Work out the finished part from the listing and answer in its coordinate system (mm). Give positions to 0.01 mm unless a question says otherwise; leave off trailing zeros. Order: outer loops, then holes, each group sorted by start corner. A loop starts at its lowest first (then second) coordinate and runs counter-clockwise, first axis right, second up. Notation, with made-up numbers: (13.25, 59.5) - (70.25, 59.5) arc R27 cw to (70.25, 76.5) - close; hole circle Ø1 at (59, 41.25). An arc over 180 degrees is marked (long way). Write each question's results on one line, items separated by ' | '.
from build123d import *

# Parameters (mm, degrees)
SKETCH1_W           = 165.75
SKETCH1_H           = 75
BOSS_EXTRUDE1_DEPTH = 3
SKETCH2_W           = 151.75
SKETCH2_H           = 5
CUT_EXTRUDE1_DEPTH  = 183.692731916
FILLET4_R           = 1
FILLET5_R           = 1
FILLET6_R           = 1
FILLET7_R           = 1
FILLET8_R           = 1
FILLET9_R           = 1
FILLET10_R          = 1
FILLET11_R          = 1
FILLET12_R          = 1
FILLET13_R          = 1
FILLET14_R          = 1
FILLET15_R          = 1
FILLET16_R          = 1
FILLET17_R          = 1
FILLET18_R          = 1
FILLET19_R          = 1
FILLET20_R          = 1
FILLET21_R          = 1
FILLET22_R          = 1
FILLET23_R          = 1
FILLET24_R          = 1
FILLET25_R          = 1
FILLET26_R          = 1
FILLET27_R          = 1


with BuildPart() as part:
    # Sketch1 → Boss-Extrude1 (new body)
    with BuildSketch(Plane(origin=(0, 0, 0), x_dir=(1, 0, 0), z_dir=(0, 1, 0))):
        with Locations((-81.877808989, 41.393258427)):
            Rectangle(SKETCH1_W, SKETCH1_H)
    extrude(amount=BOSS_EXTRUDE1_DEPTH)

    # Sketch2 → Cut-Extrude1 (cut, through all)
    with BuildSketch(Plane(origin=(0, 3, 0), x_dir=(1, 0, 0), z_dir=(0, 1, 0))):
        with Locations((-81.877808989, 68.893258427)):
            Rectangle(SKETCH2_W, SKETCH2_H)
        with Locations((-81.877808989, 57.893258427)):
            Rectangle(SKETCH2_W, SKETCH2_H)
        with Locations((-81.877808989, 46.893258427)):
            Rectangle(SKETCH2_W, SKETCH2_H)
        with Locations((-81.877808989, 35.893258427)):
            Rectangle(SKETCH2_W, SKETCH2_H)
        with Locations((-81.877808989, 24.893258427)):
            Rectangle(SKETCH2_W, SKETCH2_H)
        with Locations((-81.877808989, 13.893258427)):
            Rectangle(SKETCH2_W, SKETCH2_H)
    extrude(amount=-CUT_EXTRUDE1_DEPTH, mode=Mode.SUBTRACT)

    # Fillet4
    fillet4_edges = [part.edges().sort_by_distance(p)[0] for p in [
        (-81.877808989, 3, -60.393258427),
    ]]
    fillet(fillet4_edges, radius=FILLET4_R)

    # Fillet5
    fillet5_edges = [part.edges().sort_by_distance(p)[0] for p in [
        (-81.877808989, 3, -66.393258427),
    ]]
    fillet(fillet5_edges, radius=FILLET5_R)

    # Fillet6
    fillet6_edges = [part.edges().sort_by_distance(p)[0] for p in [
        (-81.877808989, 3, -49.393258427),
    ]]
    fillet(fillet6_edges, radius=FILLET6_R)

    # Fillet7
    fillet7_edges = [part.edges().sort_by_distance(p)[0] for p in [
        (-81.877808989, 3, -55.393258427),
    ]]
    fillet(fillet7_edges, radius=FILLET7_R)

    # Fillet8
    fillet8_edges = [part.edges().sort_by_distance(p)[0] for p in [
        (-81.877808989, 3, -38.393258427),
    ]]
    fillet(fillet8_edges, radius=FILLET8_R)

    # Fillet9
    fillet9_edges = [part.edges().sort_by_distance(p)[0] for p in [
        (-81.877808989, 3, -44.393258427),
    ]]
    fillet(fillet9_edges, radius=FILLET9_R)

    # Fillet10
    fillet10_edges = [part.edges().sort_by_distance(p)[0] for p in [
        (-81.877808989, 3, -33.393258427),
    ]]
    fillet(fillet10_edges, radius=FILLET10_R)

    # Fillet11
    fillet11_edges = [part.edges().sort_by_distance(p)[0] for p in [
        (-81.877808989, 3, -27.393258427),
    ]]
    fillet(fillet11_edges, radius=FILLET11_R)

    # Fillet12
    fillet12_edges = [part.edges().sort_by_distance(p)[0] for p in [
        (-81.877808989, 3, -22.393258427),
    ]]
    fillet(fillet12_edges, radius=FILLET12_R)

    # Fillet13
    fillet13_edges = [part.edges().sort_by_distance(p)[0] for p in [
        (-81.877808989, 3, -16.393258427),
    ]]
    fillet(fillet13_edges, radius=FILLET13_R)

    # Fillet14
    fillet14_edges = [part.edges().sort_by_distance(p)[0] for p in [
        (-81.877808989, 3, -11.393258427),
    ]]
    fillet(fillet14_edges, radius=FILLET14_R)

    # Fillet15
    fillet15_edges = [part.edges().sort_by_distance(p)[0] for p in [
        (-81.877808989, 3, -71.393258427),
    ]]
    fillet(fillet15_edges, radius=FILLET15_R)

    # Fillet16
    fillet16_edges = [part.edges().sort_by_distance(p)[0] for p in [
        (-157.752808989, 3, -68.893258427),
    ]]
    fillet(fillet16_edges, radius=FILLET16_R)

    # Fillet17
    fillet17_edges = [part.edges().sort_by_distance(p)[0] for p in [
        (-157.752808989, 3, -57.893258427),
    ]]
    fillet(fillet17_edges, radius=FILLET17_R)

    # Fillet18
    fillet18_edges = [part.edges().sort_by_distance(p)[0] for p in [
        (-157.752808989, 3, -46.893258427),
    ]]
    fillet(fillet18_edges, radius=FILLET18_R)

    # Fillet19
    fillet19_edges = [part.edges().sort_by_distance(p)[0] for p in [
        (-157.752808989, 3, -35.893258427),
    ]]
    fillet(fillet19_edges, radius=FILLET19_R)

    # Fillet20
    fillet20_edges = [part.edges().sort_by_distance(p)[0] for p in [
        (-157.752808989, 3, -24.893258427),
    ]]
    fillet(fillet20_edges, radius=FILLET20_R)

    # Fillet21
    fillet21_edges = [part.edges().sort_by_distance(p)[0] for p in [
        (-157.752808989, 3, -13.893258427),
    ]]
    fillet(fillet21_edges, radius=FILLET21_R)

    # Fillet22
    fillet22_edges = [part.edges().sort_by_distance(p)[0] for p in [
        (-6.002808989, 3, -13.893258427),
    ]]
    fillet(fillet22_edges, radius=FILLET22_R)

    # Fillet23
    fillet23_edges = [part.edges().sort_by_distance(p)[0] for p in [
        (-6.002808989, 3, -24.893258427),
    ]]
    fillet(fillet23_edges, radius=FILLET23_R)

    # Fillet24
    fillet24_edges = [part.edges().sort_by_distance(p)[0] for p in [
        (-6.002808989, 3, -35.893258427),
    ]]
    fillet(fillet24_edges, radius=FILLET24_R)

    # Fillet25
    fillet25_edges = [part.edges().sort_by_distance(p)[0] for p in [
        (-6.002808989, 3, -46.893258427),
    ]]
    fillet(fillet25_edges, radius=FILLET25_R)

    # Fillet26
    fillet26_edges = [part.edges().sort_by_distance(p)[0] for p in [
        (-6.002808989, 3, -57.893258427),
    ]]
    fillet(fillet26_edges, radius=FILLET26_R)

    # Fillet27
    fillet27_edges = [part.edges().sort_by_distance(p)[0] for p in [
        (-6.002808989, 3, -68.893258427),
    ]]
    fillet(fillet27_edges, radius=FILLET27_R)


solid = part.part
1. A cutting plane is placed at A-A, the plane z = -24. Write down the section's boundary in (x, y).
Answer list:
outline: (-164.75, 0) - (-157.75, 0) - (-157.75, 2) arc R1 ccw to (-158.75, 3) - (-164.75, 3) - close; (-6, 0) - (1, 0) - (1, 3) - (-5, 3) arc R1 ccw to (-6, 2) - close
2. Given P1, Ø1.5, axis at x = -79, z = -16, coming from the -Y side; P2, Ø6, axis at x = -59, z = -47, coming from the +Y side, each flat-ended and moving along its own axis, determine where each tip first touches the part or whether it passes through.
Answer list:
P1: y = 0 | P2: y = 2.92
3. Straight lines are drawn through the part: line 1 (X direction, y = 1.2, z = -49); line 2 (X direction, y = 2.6, z = -34); line 3 (Y direction, x = -5.5, z = -65.5). For each, find the intervals that lie inside material, in ascending order. Write a range as [from, to].
Answer list:
line 1: [-164.75, -157.75], [-6, 1] | line 2: [-164.75, -157.95], [-5.8, 1] | line 3: [0, 2.99]
4. A cutting plane is placed at B-B, the plane y = 1.3. Write down the section's boundary in (x, z).
Answer list:
outline: (-164.75, -78.89) - (1, -78.89) - (1, -3.89) - (-164.75, -3.89) - close; hole (-157.75, -71.39) - (-6, -71.39) - (-6, -66.39) - (-157.75, -66.39) - close; hole (-157.75, -60.39) - (-6, -60.39) - (-6, -55.39) - (-157.75, -55.39) - close; hole (-157.75, -49.39) - (-6, -49.39) - (-6, -44.39) - (-157.75, -44.39) - close; hole (-157.75, -38.39) - (-6, -38.39) - (-6, -33.39) - (-157.75, -33.39) - close; hole (-157.75, -27.39) - (-6, -27.39) - (-6, -22.39) - (-157.75, -22.39) - close; hole (-157.75, -16.39) - (-6, -16.39) - (-6, -11.39) - (-157.75, -11.39) - close
5. A cutting plane is placed at C-C, the plane x = -49. State how many separate pieces and enclosed holes the cut face has, then the cut area to 3 significant figures.
Answer list:
separate pieces: 7 | enclosed holes: 0 | area: 132 mm^2
